from build123d import *

# Parameters (mm, degrees)
F0_W     = 750
F0_H     = 750
F0_W_2   = 550
F0_H_2   = 550
F1_DEPTH = 100
F3_DEPTH = 100


with BuildPart() as f1:
    # F0 (on Top) → F1 (new body)
    with BuildSketch(Plane.XY):
        with Locations((244.376540184, 327.9930502176)):
            Rectangle(F0_W, F0_H)
        with Locations((244.376540184, 327.9930502176)):
            Rectangle(F0_W_2, F0_H_2, mode=Mode.SUBTRACT)
    extrude(amount=F1_DEPTH)

    # F2 (on face) → F3 (join)
    with BuildSketch(Plane.XZ.offset(47.0069497824)):
        with BuildLine():
            Line((244.376540184, 50), (254.376540184, 50))
            ThreePointArc((254.376540184, 50), (251.4476079959, 57.0710678119), (244.376540184, 60))
            Line((244.376540184, 60), (244.376540184, 50))
        make_face()
        with BuildLine():
            Line((234.376540184, 50), (244.376540184, 50))
            Line((244.376540184, 50), (244.376540184, 60))
            ThreePointArc((244.376540184, 60), (237.3054723722, 57.0710678119), (234.376540184, 50))
        make_face()
        with BuildLine():
            Line((244.376540184, 40), (244.376540184, 50))
            Line((244.376540184, 50), (234.376540184, 50))
            ThreePointArc((234.376540184, 50), (237.3054723722, 42.9289321881), (244.376540184, 40))
        make_face()
        with BuildLine():
            ThreePointArc((244.376540184, 40), (251.4476079959, 42.9289321881), (254.376540184, 50))
            Line((254.376540184, 50), (244.376540184, 50))
            Line((244.376540184, 50), (244.376540184, 40))
        make_face()
    extrude(amount=F3_DEPTH)


solid = f1.part
Can you work these out from the model? Positions are in its coordinate system, mm. A direction names the side the tool comes from. Give positions to 0.01 mm unless a question says otherwise; leave off trailing zeros. Loops run counter-clockwise (first coordinate to the right, second up) from the corner with the lowest first, then second, coordinate; pieces in that order, holes last. Notation, with made-up numbers: M -30.5,34.25 L 11.5,34.25 A19 cw 11.5,62.25 Z; hole C 30,18 d9. An arc over 180 degrees is marked long. One line per item, written item: value. Start each with the question number.
1) If we section it at C-C, the plane z = 88.5: Write out the boundary of the cut face in (x, y), and give its area (3 significant figures).
2) If we section it at A-A, the plane y = 258.5: Write out the boundary of the cut face in (x, z), and give its area (3 significant figures).
3) On a 3-axis mill with a long thin cutter (end or side, diameter ignored), from which of +Z, -Z, +X, -X, +Y, -Y can I reach the whole of each face in a straight line? I mean faces 4 (the face through (241, 602.993, 49)), 5 (the face through (-130.623, 323, 49)). Say none if no direction works.
4) I'm going to push a flat-ended pin straight in: pin 1 (5 mm diameter, centred on x = 153.5, z = 19.5, fed in from -Y). Where does the tip first touch, or does it pass through?
5) If I drill on line 1 (X direction, y = 103, z = 18); line 2 (Y direction, x = 346.5, z = 75); line 3 (Y direction, x = 521, z = 61), over which ranges is the centre line in solid material (lowest first)? Write a range as [from, to].
6) If we section it at B-B, the plane x = 10: Write out the boundary of the cut face in (y, z).
7) Thinking about a two-plate mould opening in Y: for faces 1 (the face through (241, 52.993, 49)), 2 (the face through (244, -147.007, 50)), 3 (the face through (619.377, 323, 49)), which applies, +Y half, -Y half, draft (parallel to the pull), parting line (faces both ways), or undercut?
Completed:
1. outline: M -130.62,-47.01 L 619.38,-47.01 L 619.38,702.99 L -130.62,702.99 Z; hole M -30.62,52.99 L 519.38,52.99 L 519.38,602.99 L -30.62,602.99 Z
1. area: 260,000 mm^2
2. outline: M -130.62,0 L -30.62,0 L -30.62,100 L -130.62,100 Z; M 519.38,0 L 619.38,0 L 619.38,100 L 519.38,100 Z
2. area: 20,000 mm^2
3. face 4: +Z, -Z
3. face 5: +Z, -Z, -X, +Y, -Y
4. pin 1: stops at y = -47.01
5. line 1: x = [-130.62, -30.62], [519.38, 619.38]
5. line 2: y = [-47.01, 52.99], [602.99, 702.99]
5. line 3: y = [-47.01, 702.99]
6. outline: M -47.01,0 L 52.99,0 L 52.99,100 L -47.01,100 Z; M 602.99,0 L 702.99,0 L 702.99,100 L 602.99,100 Z
7. face 1: undercut
7. face 2: -Y half
7. face 3: draft
